Work out the finished part from the listing and answer in its coordinate system (mm). A direction names the side the tool comes from. Round coordinates to 2 decimals unless told otherwise and drop trailing zeros. Write each loop counter-clockwise with the first axis right and the second up, starting at its lowest first coordinate (ties: lowest second). Pieces come first, ordered by that corner, then holes.
1. Find section D-D (z = 87). Write down the section's boundary in (x, y), and give its area (3 significant figures).
2. Straight lines are drawn through the part: probe 1 along Y at (x, z) = (-122, 131); probe 2 along X at (y, z) = (-21, 22); probe 3 along Z at (x, y) = (-16.5, -40). For each, find the intervals that lie inside material, in ascending order.
3. Determine the mould class of faces 4 (the face through (-39.21, -21.57, 36.67)), 5 (the face through (-15, -7, 75)), 6 (the face through (-80, -15, 101)) for opening direction Y: pulls with the +Y half, pulls with the -Y half, needs draft (parallel to the pull), parting line crosses it, or undercut.
4. Find section B-B (z = 31.5). Write down the section's boundary in (x, y), and give its area (3 significant figures).
5. Find section A-A (x = -87.5). Write down the section's boundary in (y, z).
6. A tool of negligible diameter and unlimited length cuts with its end or side. For faces 1 (the face through (-130, -7, 101)), 2 (the face through (-30, -7, 125)), 3 (the face through (-106, -28.4, 23.7)), from which of +Z, -Z, +X, -X, +Y, -Y can it reach the whole face along a straight path? Write none if from no direction.
7. Find section C-C (x = -52.5). Write down the section's boundary in (y, z).
8. Flat-ended cylindrical pins translate along their axes: pin 1 Ø6.5 at (x, y) = (-107.32, -24.19) entering from +Z; pin 2 Ø1 at (x, y) = (-52, -32) entering from +Z; pin 3 Ø6 at (x, y) = (-43, -20.5) entering from -Z; pin 4 Ø10.5 at (x, y) = (-107, -21.5) entering from -Z. Find the tip coordinate at first contact, or state that the pin passes through.
```python
from build123d import *

# Parameters (mm, degrees)
F0_R     = 4.7966354506
F0_R_2   = 4.3722617323
F1_DEPTH = 15
F2_DEPTH = 50
F3_R     = 3.9330231178
F3_R_2   = 4.374414862
F3_R_3   = 4.2015516797
F3_R_4   = 3.7245553563
F3_R_5   = 3.5273482247
F4_DEPTH = 69
F3_R_6   = 6.4374509429
F3_R_7   = 5.9942154244
F5_DEPTH = 23.7


with BuildPart() as f1:
    # F0 (on Front) → F1 (new body)
    with BuildSketch(Plane.XZ):
        Polygon((-130, 50), (-100, 50), (-30, 50), (-30, 100), (-30, 150), (-130, 150), align=None)
        with Locations((-113.601192832, 138.8020068407)):
            Circle(F0_R, mode=Mode.SUBTRACT)
        with Locations((-45.5297119915, 138.8020068407)):
            Circle(F0_R_2, mode=Mode.SUBTRACT)
        Polygon((-30, 50), (0, 50), (-30, 100), align=None)
    extrude(amount=F1_DEPTH)

    # F0 (on Front) → F2 (join)
    with BuildSketch(Plane.XZ):
        Polygon((-130, 50), (-100, 0), (-100, 50), align=None)
        Polygon((-100, 0), (0, 0), (0, 50), (-30, 50), (-100, 50), align=None)
    extrude(amount=F2_DEPTH)

    # F3 (on Top) → F4 (cut)
    with BuildSketch(Plane.XY):
        with Locations((-20.6890981644, -24.4208239019)):
            Circle(F3_R)
        with Locations((-86.1961916089, -24.0469053388)):
            Circle(F3_R_2)
        with Locations((-107.3154211044, -24.1862814873)):
            Circle(F3_R_3)
        with Locations((-42.7642799914, -22.6896554232)):
            Circle(F3_R_4)
        with Locations((-7.7202138491, -41.0906225443)):
            Circle(F3_R_5)
    extrude(amount=F4_DEPTH, mode=Mode.SUBTRACT)

    # F3 (on Top) → F5 (cut)
    with BuildSketch(Plane.XY):
        with Locations((-107.3154211044, -24.1862814873)):
            Circle(F3_R_6)
        with Locations((-107.3154211044, -24.1862814873)):
            Circle(F3_R_3, mode=Mode.SUBTRACT)
        with Locations((-42.7642799914, -22.6896554232)):
            Circle(F3_R_7)
        with Locations((-42.7642799914, -22.6896554232)):
            Circle(F3_R_4, mode=Mode.SUBTRACT)
    extrude(amount=F5_DEPTH, mode=Mode.SUBTRACT)


solid = f1.part
```
Worked answers:
1. outline: (-130, -15) - (-22.2, -15) - (-22.2, 0) - (-130, 0) - close
1. area: 1,620 mm2
2. probe 1: y = -15 to 0
2. probe 2: x = -113.2 to -112.91, -101.72 to -89.33, -83.06 to -48.52, -37.01 to -22.63, -18.75 to 0
2. probe 3: z = 0 to 50
3. face 4: undercut
3. face 5: needs draft
3. face 6: pulls with the -Y half
4. outline: (-118.9, -50) - (0, -50) - (0, 0) - (-118.9, 0) - close; hole circle Ø8.4 at (-107.32, -24.19); hole circle Ø8.75 at (-86.2, -24.05); hole circle Ø7.45 at (-42.76, -22.69); hole circle Ø7.87 at (-20.69, -24.42); hole circle Ø7.05 at (-7.72, -41.09)
4. area: 5,700 mm2
5. outline: (-50, 0) - (-28.22, 0) - (-28.22, 50) - (-50, 50) - close; (-19.87, 0) - (0, 0) - (0, 150) - (-15, 150) - (-15, 50) - (-19.87, 50) - close
6. face 1: +Z, -Z, -X, +Y, -Y
6. face 2: +Z, +X, +Y, -Y
6. face 3: -Z
7. outline: (-50, 0) - (0, 0) - (0, 150) - (-15, 150) - (-15, 50) - (-50, 50) - close
8. pin 1: passes through
8. pin 2: stops at z = 50
8. pin 3: stops at z = 23.7
8. pin 4: stops at z = 2.98
